Verification items for the finished model (mm, model axes). A direction names the side the tool comes from. Give positions to 0.01 mm unless a question says otherwise; leave off trailing zeros. Write each loop counter-clockwise with the first axis right and the second up, starting at its lowest first coordinate (ties: lowest second). Pieces come first, ordered by that corner, then holes. Notation, with made-up numbers: (76, -25.75) -> (122, -25.75) arc R23 ccw to (122, -12.75) -> close; hole circle Ø7 at (-11, 71.5). An arc over 180 degrees is marked (long way). Answer as CSV lines item,"result". Start each with the question number.
1) Mould release check, pull along X, two halves, no side actions. Record for faces 5 (the flat face through (0.242, 157, 19)), 6 (the cylindrical face through (0, 81.52, 20.05)), 7 (the flat face through (0, 149, 8.477)): released by +X, released by -X, zero draft, split by the parting line, or undercut.
2) Tool access check on faces 1 (the flat face through (0, 149, 9.972)), 2 (the flat face through (0, 165.354, 15)), 3 (the flat face through (0, 49, 9.999)), 4 (the flat face through (-0.273, 157, 19)). Record the directions out of +Z, -Z, +X, -X, +Y, -Y that give a thin tool (end or side, any length) a straight path to the whole face; none if there is none.
3) Gauge pin test, flat ends, axial feed: pin 1 Ø1.5 at (x, y) = (-2.5, 91.5) entering from +Z; pin 2 Ø1.5 at (x, y) = (2, 29.5) entering from -Z; pin 3 Ø1.4 at (y, z) = (160, 19) entering from -X. Record the tip position at first contact, or that the pin passes through.
4) Sectioned sample at B-B on x = -2.25. Record the cut outline in (y, z).
5) Material ranges on L1, parallel to Z at x = -1, y = 45.5; L2, parallel to Y at x = 1.5, z = 9.5; L3, parallel to Z at x = -2, y = 53, recorded low to high.
```python
from build123d import *

# Parameters (mm, degrees)
F0_W     = 7.450324
F0_H     = 16.439302
F1_DEPTH = 165.354
F3_W     = 50.933755
F3_H     = 1.793447
F4_DEPTH = 232.41
F6_W     = 0.515365
F6_H     = 3.407134
F7_DEPTH = 43.6118
F8_W     = 37.184134
F8_H     = 1.494539
F9_DEPTH = 232.41


with BuildPart() as f1:
    # F0 (on Front) → F1 (new body)
    with BuildSketch(Plane.XZ):
        with BuildLine():
            Line((-3.806144, 16.439302), (3.64418, 16.439302))
            ThreePointArc((3.64418, 16.439302), (-0.080982, 20.048889), (-3.806144, 16.439302))
        make_face()
        with Locations((-0.080982, 8.219651)):
            Rectangle(F0_W, F0_H)
        with BuildLine():
            ThreePointArc((-3.806144, 0), (-0.080982, -3.725162), (3.64418, 0))
            Line((3.64418, 0), (-3.806144, 0))
        make_face()
    extrude(amount=-F1_DEPTH)

    # F3 (on offset) → F4 (cut)
    with BuildSketch(Plane.YZ.offset(139.7)):
        with BuildLine():
            Line((23.742341, 8.20523), (23.742341, 9.998677))
            ThreePointArc((23.742341, 9.998677), (23.042202, 9.101954), (23.742341, 8.20523))
        make_face()
        with Locations((49.209218, 9.101954)):
            Rectangle(F3_W, F3_H)
    extrude(amount=-F4_DEPTH, mode=Mode.SUBTRACT)

    # F6 (on offset) → F7 (cut)
    with BuildSketch(Plane.XZ.offset(-149.352)):
        with Locations((-0.015719, 18.905162)):
            Rectangle(F6_W, F6_H)
    extrude(amount=-F7_DEPTH, mode=Mode.SUBTRACT)

    # F8 (on offset) → F9 (cut)
    with BuildSketch(Plane.YZ.offset(139.7)):
        with Locations((151.09729, 9.224657)):
            Rectangle(F8_W, F8_H)
    extrude(amount=-F9_DEPTH, mode=Mode.SUBTRACT)


solid = f1.part
```
Ans:
1,face 5,"undercut"
1,face 6,"split by the parting line"
1,face 7,"zero draft"
2,face 1,"+X, -X, +Y"
2,face 2,"+Z, -Z, +X, -X, +Y"
2,face 3,"+X, -X"
2,face 4,"+Z, +Y"
3,pin 1,"stops at z = 19.65"
3,pin 2,"stops at z = -3.48"
3,pin 3,"stops at x = -3.24"
4,outline,"(0, -3.03) -> (165.35, -3.03) -> (165.35, 8.48) -> (132.51, 8.48) -> (132.51, 9.97) -> (165.35, 9.97) -> (165.35, 19.35) -> (0, 19.35) -> close; hole (23.74, 8.21) -> (74.68, 8.21) -> (74.68, 10) -> (23.74, 10) arc R0.92 ccw to start"
5,L1,"z = -3.61 to 8.21, 10 to 19.93"
5,L2,"y = 0 to 23.13, 74.68 to 132.51"
5,L3,"z = -3.19 to 8.21, 10 to 19.52"
